Work out the finished part from the listing and answer in its coordinate system (mm). Face numbers are marked on the shaded views. Round coordinates to 2 decimals unless told otherwise and drop trailing zeros. Order: outer loops, then holes, each group sorted by start corner. A loop starts at its lowest first (then second) coordinate and runs counter-clockwise, first axis right, second up. Notation, with made-up numbers: M -36,45 L 13,45 A21 cw 13,63 Z; hole C 37,-34 d8. An arc over 180 degrees is marked long. Return JSON: item names as keys, results as strings.
from build123d import *

# Parameters (mm, degrees)
F0_W     = 48
F0_H     = 8
F1_DEPTH = 5
F2_W     = 48
F2_H     = 5
F3_DEPTH = 3.5
F4_R     = 3


with BuildPart() as f1:
    # F0 (on Top) → F1 (new body)
    with BuildSketch(Plane.XY):
        Rectangle(F0_W, F0_H)
    extrude(amount=F1_DEPTH)

    # F2 (on face) → F3 (cut)
    with BuildSketch(Plane.XY.offset(5)):
        Rectangle(F2_W, F2_H)
    extrude(amount=-F3_DEPTH, mode=Mode.SUBTRACT)

    # F4
    f4_edges = [f1.edges().sort_by_distance(p)[0] for p in [
        (0, -4, 0),
        (0, 4, 0),
    ]]
    fillet(f4_edges, radius=F4_R)


solid = f1.part
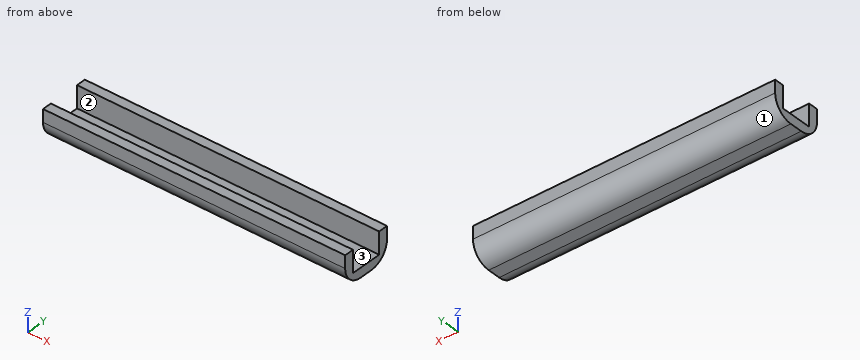
Item 1: Find section C-C (y = -0.5). Determine the outline of the cut face in (x, z), plus the area to 3 significant figures.
Output:
{"outline": "M -24,0 L 24,0 L 24,1.5 L -24,1.5 Z", "area": "72.0 mm^2"}
Item 2: Consider line 1 along Y through (x, z) = (-4, 4.65); line 2 along Y through (x, z) = (9.5, 2.35); line 3 along Z through (x, y) = (7.5, -0.25). Determine where each line is inside the solid, lowest interval first. Write a range as [from, to].
Output:
{"line 1": "y = [-4, -2.5], [2.5, 4]", "line 2": "y = [-3.93, -2.5], [2.5, 3.93]", "line 3": "z = [0, 1.5]"}
Item 3: Find section A-A (z = 3.9). Determine the outline of the cut face in (x, y), plus the area to 3 significant figures.
Output:
{"outline": "M -24,-4 L 24,-4 L 24,-2.5 L -24,-2.5 Z; M -24,2.5 L 24,2.5 L 24,4 L -24,4 Z", "area": "144 mm^2"}
Item 4: The mould has two halves that part along Y. Classify the marked faces 1, 2 and 3: pulls with the +Y half, pulls with the -Y half, needs draft (parallel to the pull), parting line crosses it, or undercut.
Output:
{"face 1": "pulls with the +Y half", "face 2": "undercut", "face 3": "undercut"}
Item 5: Find section B-B (x = -4.5). Determine the outline of the cut face in (y, z).
Output:
{"outline": "M -4,3 A3 ccw -1,0 L 1,0 A3 ccw 4,3 L 4,5 L 2.5,5 L 2.5,1.5 L -2.5,1.5 L -2.5,5 L -4,5 Z"}
Item 6: Find section D-D (z = 2). Determine the outline of the cut face in (x, y).
Output:
{"outline": "M -24,-3.83 L 24,-3.83 L 24,-2.5 L -24,-2.5 Z; M -24,2.5 L 24,2.5 L 24,3.83 L -24,3.83 Z"}
Item 7: Each of these flat-tipped pins is pushed along its axis until it touches: pin 1 (1.5 mm diameter, centred on y = 2, z = 2, fed in from -X); pin 2 (2 mm diameter, centred on x = -13, y = 3, fed in from -Z). Where does it stop, or does it pass through?
Output:
{"pin 1": "stops at x = -24", "pin 2": "stops at z = 0.17"}
